```python
from build123d import *

# Parameters (mm, degrees)
F0_R     = 50
F0_R_2   = 45
F1_DEPTH = 100
F0_R_3   = 40
F2_DEPTH = 5
F3_R     = 13.8817279836
F4_DEPTH = 50


with BuildPart() as f1:
    # F0 (on Top) → F1 (new body)
    with BuildSketch(Plane.XY):
        Circle(F0_R)
        Circle(F0_R_2, mode=Mode.SUBTRACT)
    extrude(amount=F1_DEPTH)

    # F0 (on Top) → F2 (join)
    with BuildSketch(Plane.XY):
        Circle(F0_R)
        Circle(F0_R_2, mode=Mode.SUBTRACT)
        Circle(F0_R_2)
        Circle(F0_R_3, mode=Mode.SUBTRACT)
        Circle(F0_R_3)
    extrude(amount=-F2_DEPTH)

    # F3
    f3_edges = [f1.edges().sort_by_distance(p)[0] for p in [
        (-50, 0, -5),
    ]]
    fillet(f3_edges, radius=F3_R)

    # F0 (on Top) → F4 (join)
    with BuildSketch(Plane.XY):
        Circle(F0_R_2)
        Circle(F0_R_3, mode=Mode.SUBTRACT)
    extrude(amount=F4_DEPTH)


solid = f1.part
```
Part model, mm, in its own coordinate system. A direction names the side the tool comes from. Round coordinates to 2 decimals unless told otherwise and drop trailing zeros. Loops run counter-clockwise (first coordinate to the right, second up) from the corner with the lowest first, then second, coordinate; pieces in that order, holes last. Notation, with made-up numbers: (11, 52) -> (30, 52) arc R23 cw to (30, 85) -> close; hole circle Ø1 at (36.5, 48). An arc over 180 degrees is marked (long way). Use CSV: the item, a comma, the result in double quotes. Start each with the question number.
1) Cut at D-D, the plane z = 55. Write the cut outline in (x, y).
2) Cut at A-A, the plane x = 0. Write the cut outline in (y, z).
3) Drop flat-ended pins along their axis: P1, Ø1.5, axis at y = -38.5, z = 41.5, coming from the -X side; P2, Ø4, axis at y = -12.5, z = 22.5, coming from the +X side; P3, Ø4, axis at y = 33, z = 69.5, coming from the +X side. Give the stop position or say it passes through.
4) Wall check: L1, parallel to Y at x = 0, z = 35; L2, parallel to Y at x = 0, z = 80; L3, parallel to Z at x = 12.5, y = 25. Give the ranges that are in metal, low to high. Write a range as [from, to].
5) Cut at C-C, the plane z = 21. Write the cut outline in (x, y).
6) Which spindle directions (+Z, -Z, +X, -X, +Y, -Y) get a long thin tool onto all of the face, cutting with end or side? Do faces 1 (the flat face through (-1, 1, -5)), 2 (the flat face through (-30.2, -26.5, 50)). Say none if no direction does.
Determined:
1,outline,"circle Ø100 at (0, 0); hole circle Ø90 at (0, 0)"
2,outline,"(-50, 8.88) arc R13.88 ccw to (-36.12, -5) -> (36.12, -5) arc R13.88 ccw to (50, 8.88) -> (50, 100) -> (45, 100) -> (45, 50) -> (40, 50) -> (40, 0) -> (-40, 0) -> (-40, 50) -> (-45, 50) -> (-45, 100) -> (-50, 100) -> close"
3,P1,"stops at x = -32.79"
3,P2,"stops at x = 48.89"
3,P3,"stops at x = 39.23"
4,L1,"y = [-50, -40], [40, 50]"
4,L2,"y = [-50, -45], [45, 50]"
4,L3,"z = [-5, 0]"
5,outline,"circle Ø100 at (0, 0); hole circle Ø80 at (0, 0)"
6,face 1,"-Z, +X, -X, +Y, -Y"
6,face 2,"+Z"
